Could you check a few things on this drawing? It's one solid part, dimensions in mm from its lowest x, y, z. Round coordinates to 2 decimals unless told otherwise and drop trailing zeros. Write each loop counter-clockwise with the first axis right and the second up, starting at its lowest first coordinate (ties: lowest second). Pieces come first, ordered by that corner, then holes. Notation, with made-up numbers: (-30, -21) -> (23, -21) arc R27 ccw to (23, 7) -> close; hole circle Ø9 at (72, 47.5). An arc over 180 degrees is marked (long way). Answer in a Markdown table with one row per item.
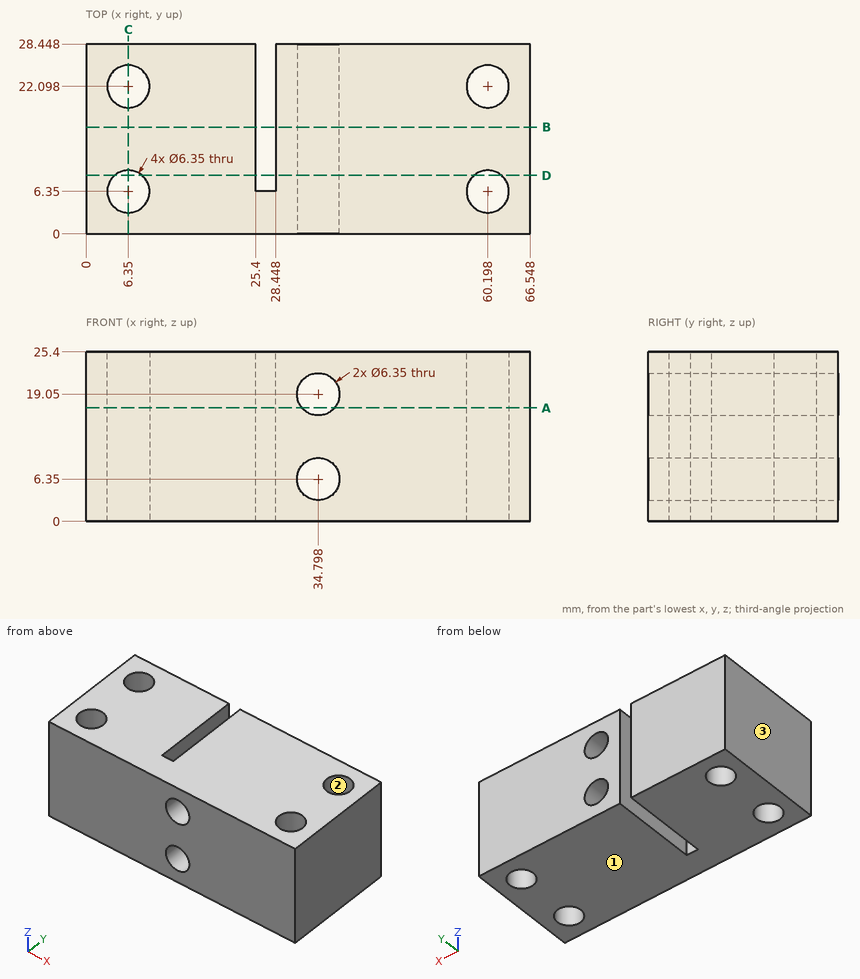
1) I want a section at C-C, the plane x = 6.35. List the corners of the cut face in (y, z) for me (3 decimals), and give its area (3 significant figures).
Response:
| item | result |
|---|---|
| outline | (0, 0) -> (3.175, 0) -> (3.175, 25.4) -> (0, 25.4) -> close; (9.525, 0) -> (18.923, 0) -> (18.923, 25.4) -> (9.525, 25.4) -> close; (25.273, 0) -> (28.448, 0) -> (28.448, 25.4) -> (25.273, 25.4) -> close |
| area | 400 mm^2 |
2) I want a section at D-D, the plane y = 8.75. List the corners of the cut face in (x, z) for me (3 decimals).
Response:
| item | result |
|---|---|
| outline | (0, 0) -> (4.271, 0) -> (4.271, 25.4) -> (0, 25.4) -> close; (8.429, 0) -> (25.4, 0) -> (25.4, 25.4) -> (8.429, 25.4) -> close; (28.448, 0) -> (58.119, 0) -> (58.119, 25.4) -> (28.448, 25.4) -> close; (62.277, 0) -> (66.548, 0) -> (66.548, 25.4) -> (62.277, 25.4) -> close; hole circle Ø6.35 at (34.798, 6.35); hole circle Ø6.35 at (34.798, 19.05) |
3) I need wall thicknesses on line 1 (X direction, y = 25.75, z = 21); line 2 (Z direction, x = 32, y = 13.5); line 3 (X direction, y = 19.25, z = 22.5). Which ranges of each line are inside material? Lowest first, please. Write a range as [from, to].
Response:
| item | result |
|---|---|
| line 1 | x = [0, 25.4], [28.45, 32.29], [37.3, 66.55] |
| line 2 | z = [0, 4.85], [7.85, 17.55], [20.55, 25.4] |
| line 3 | x = [0, 4.95], [7.75, 25.4], [28.45, 58.79], [61.6, 66.55] |
4) I want a section at B-B, the plane y = 16. List the corners of the cut face in (x, z) for me (3 decimals).
Response:
| item | result |
|---|---|
| outline | (0, 0) -> (25.4, 0) -> (25.4, 25.4) -> (0, 25.4) -> close; (28.448, 0) -> (66.548, 0) -> (66.548, 25.4) -> (28.448, 25.4) -> close; hole circle Ø6.35 at (34.798, 6.35); hole circle Ø6.35 at (34.798, 19.05) |
5) We'd pull the mould along X, two halves only. Please class the marked faces 1, 2 and 3: +X half, -X half, draft (parallel to the pull), parting line (faces both ways), or undercut.
Response:
| item | result |
|---|---|
| face 1 | draft |
| face 2 | undercut |
| face 3 | -X half |
6) I want a section at A-A, the plane z = 17. List the corners of the cut face in (x, y) for me (3 decimals).
Response:
| item | result |
|---|---|
| outline | (0, 0) -> (32.374, 0) -> (32.374, 28.448) -> (28.448, 28.448) -> (28.448, 6.35) -> (25.4, 6.35) -> (25.4, 28.448) -> (0, 28.448) -> close; (37.222, 0) -> (66.548, 0) -> (66.548, 28.448) -> (37.222, 28.448) -> close; hole circle Ø6.35 at (6.35, 6.35); hole circle Ø6.35 at (6.35, 22.098); hole circle Ø6.35 at (60.198, 6.35); hole circle Ø6.35 at (60.198, 22.098) |
7) For pin 1 (8.5 mm diameter, centred on x = 34.798, z = 19.05, fed in from +Y), with a flat end and sliding along its axis, tell me the tip position at first contact or that it passes through.
Response:
| item | result |
|---|---|
| pin 1 | stops at y = 28.45 |
